The model under review builds one solid part; all positions refer to its coordinate system, in mm. A direction names the side the tool comes from. Coordinates: 2 decimals unless noted, no trailing zeros. Order: outer loops, then holes, each group sorted by start corner. A loop starts at its lowest first (then second) coordinate and runs counter-clockwise, first axis right, second up. Notation, with made-up numbers: M 51.25,34 L 70.25,34 A4 ccw 70.25,39 Z; hole C -9.5,57 d5. An arc over 180 degrees is marked long. Answer as CSV lines item,"result". Start each with the question number.
Q1. Consider section A-A on x = 0. Write out the cut boundary in (y, z).
Q2. Machinability: for faces 1 (the face through (-0.54, -5.18, -2.44)), 2 (the face through (0, -7, 0)), which of the approach directions +Z, -Z, +X, -X, +Y, -Y give a long, thin tool a straight path to every point of the face, cutting with its end or side? Answer none if there is none.
Q3. Wall thickness on L1, parallel to Y at x = 2.5, z = 0.75; L2, parallel to Y at x = 2, z = -1.25; L3, parallel to Z at x = -2, y = -3.5: over which ranges is each line inside the solid? List them lowest first. Write a range as [from, to].
Q4. Consider section D-D on y = -6. Write out the cut boundary in (x, z).
Q5. Consider section C-C on y = -0.75. Write out the cut boundary in (x, z).
Q6. For P1, Ø4, axis at y = -5.5, z = -3, coming from the +X side; P2, Ø1, axis at y = -4, z = -3, coming from the +X side; P3, Ø2, axis at x = -2.5, y = -2, coming from the -Z side; P4, Ø3, axis at x = 2, z = -2, coming from the -Y side, all flat-tipped, find the tip position at first contact; note any pin that passes through.
Q7. Consider section B-B on z = 0. Write out the cut boundary in (x, y), and give its area (3 significant figures).
from build123d import *

# Parameters (mm, degrees)
F0_R     = 1.65
F1_DEPTH = 7
F0_R_2   = 2.5
F2_DEPTH = 7
F0_R_3   = 4
F3_DEPTH = 4
F4_R     = 0.6


with BuildPart() as f1:
    # F0 (on Front) → F1 (new body)
    with BuildSketch(Plane.XZ):
        Circle(F0_R)
    extrude(amount=F1_DEPTH)

    # F0 (on Front) → F2 (join)
    with BuildSketch(Plane.XZ):
        Circle(F0_R_2)
        Circle(F0_R, mode=Mode.SUBTRACT)
    extrude(amount=F2_DEPTH)

    # F0 (on Front) → F3 (join)
    with BuildSketch(Plane.XZ):
        Circle(F0_R_3)
        Circle(F0_R_2, mode=Mode.SUBTRACT)
    extrude(amount=F3_DEPTH)

    # F4
    f4_edges = [f1.edges().sort_by_distance(p)[0] for p in [
        (-2.5, -7, 0),
    ]]
    fillet(f4_edges, radius=F4_R)


solid = f1.part
Evaluation:
1,outline,"M -7,-1.9 A0.6 ccw -6.4,-2.5 L -4,-2.5 L -4,-4 L 0,-4 L 0,4 L -4,4 L -4,2.5 L -6.4,2.5 A0.6 ccw -7,1.9 Z"
2,face 1,"-Y"
2,face 2,"+Z, -Z, +X, -X, -Y"
3,L1,"y = [-4, 0]"
3,L2,"y = [-6.79, 0]"
3,L3,"z = [-3.46, 3.46]"
4,outline,"C 0,0 d5"
5,outline,"C 0,0 d8"
6,P1,"stops at x = 3.63"
6,P2,"stops at x = 3.12"
6,P3,"stops at z = -3.71"
6,P4,"stops at y = -7"
7,outline,"M -4,-4 L -2.5,-4 L -2.5,-6.4 A0.6 ccw -1.9,-7 L 1.9,-7 A0.6 ccw 2.5,-6.4 L 2.5,-4 L 4,-4 L 4,0 L -4,0 Z"
7,area,"46.8 mm²"
